Read the model definition and answer for the solid it produces. Units are mm, in the model's axes. A direction names the side the tool comes from. Give positions to 0.01 mm unless a question says otherwise; leave off trailing zeros. Order: outer loops, then holes, each group sorted by start corner. A loop starts at its lowest first (then second) coordinate and runs counter-clockwise, first axis right, second up. Notation, with made-up numbers: (58.5, 23.25) - (87.5, 23.25) arc R16 cw to (87.5, 37.25) - close; hole circle Ø3 at (85.25, 78.5). An arc over 180 degrees is marked (long way). Return JSON: item names as keys, results as strings.
Autodesk Inventor part; units mm, degrees
ref_plane "YZ Plane" through (0, 0, 0) normal (1, 0, 0) x (0, 1, 0)
ref_plane "XZ Plane" through (0, 0, 0) normal (0, 1, 0) x (-1, 0, 0)
ref_plane "XY Plane" through (0, 0, 0) normal (0, 0, 1) x (1, 0, 0)
sketch "스케치1" plane through (0, 0, 0) normal (0, 0, 1) x (1, 0, 0)
  line L0 (15, -15) -> (-15, -15)
  line L1 (-15, -15) -> (-15, 15)
  line L2 (-15, 15) -> (15, 15)
  line L3 (15, 15) -> (15, -15)
  circle A0 centre (0, 0) radius 2.5
  line L4 (-3.15, -15) -> (3.15, -15)
  line L5 (-4.15, -15) -> (4.15, -15)
  line L6 (3.15, -15) -> (3.15, -12.5)
  line L7 (-3.15, -12.5) -> (-3.15, -15)
  line L8 (-5.5, -12.5) -> (5.5, -12.5)
  line L9 (5.5, -12.5) -> (5.5, -6.9)
  line L10 (-5.5, -6.9) -> (-5.5, -12.5)
  line L11 (-5.5, -6.9) -> (-3, -4.4)
  line L12 (5.5, -6.9) -> (3, -4.4)
  line L13 (-3, -4.4) -> (3, -4.4)
  line L14 (-13.25, -13.25) -> (-7.25, -13.25)
  line L15 (-7.25, -13.25) -> (-7.25, -7.25)
  line L16 (-7.25, -7.25) -> (-13.25, -7.25)
  line L17 (-13.25, -7.25) -> (-13.25, -13.25)
  line L18 (0, 0) -> (-1, 0)
  line L19 (0, 0) -> (0, -1)
  line L20 (13.25, -13.25) -> (7.25, -13.25)
  line L21 (7.25, -13.25) -> (7.25, -7.25)
  line L22 (7.25, -7.25) -> (13.25, -7.25)
  line L23 (13.25, -7.25) -> (13.25, -13.25)
  line L24 (-13.25, 13.25) -> (-7.25, 13.25)
  line L25 (-7.25, 13.25) -> (-7.25, 7.25)
  line L26 (-7.25, 7.25) -> (-13.25, 7.25)
  line L27 (-13.25, 7.25) -> (-13.25, 13.25)
  line L28 (13.25, 7.25) -> (13.25, 13.25)
  line L29 (13.25, 13.25) -> (7.25, 13.25)
  line L30 (7.25, 13.25) -> (7.25, 7.25)
  line L31 (7.25, 7.25) -> (13.25, 7.25)
  line L32 (6.9, 5.5) -> (4.4, 3)
  line L33 (12.5, 5.5) -> (6.9, 5.5)
  line L34 (15, -3.15) -> (15, 3.15)
  line L35 (15, -4.15) -> (15, 4.15)
  line L36 (15, 3.15) -> (12.5, 3.15)
  line L37 (12.5, -3.15) -> (15, -3.15)
  line L38 (12.5, -5.5) -> (12.5, 5.5)
  line L39 (6.9, -5.5) -> (12.5, -5.5)
  line L40 (4.4, -3) -> (4.4, 3)
  line L41 (6.9, -5.5) -> (4.4, -3)
  line L42 (-5.5, 6.9) -> (-3, 4.4)
  line L43 (-5.5, 12.5) -> (-5.5, 6.9)
  line L44 (3.15, 15) -> (-3.15, 15)
  line L45 (4.15, 15) -> (-4.15, 15)
  line L46 (-3.15, 15) -> (-3.15, 12.5)
  line L47 (3.15, 12.5) -> (3.15, 15)
  line L48 (5.5, 12.5) -> (-5.5, 12.5)
  line L49 (5.5, 6.9) -> (5.5, 12.5)
  line L50 (3, 4.4) -> (-3, 4.4)
  line L51 (5.5, 6.9) -> (3, 4.4)
  line L52 (-6.9, -5.5) -> (-4.4, -3)
  line L53 (-12.5, -5.5) -> (-6.9, -5.5)
  line L54 (-15, 3.15) -> (-15, -3.15)
  line L55 (-15, 4.15) -> (-15, -4.15)
  line L56 (-15, -3.15) -> (-12.5, -3.15)
  line L57 (-12.5, 3.15) -> (-15, 3.15)
  line L58 (-12.5, 5.5) -> (-12.5, -5.5)
  line L59 (-6.9, 5.5) -> (-12.5, 5.5)
  line L60 (-4.4, 3) -> (-4.4, -3)
  line L61 (-6.9, 5.5) -> (-4.4, 3)
  dimension "d0" = 30
  dimension "d1" = 30
  dimension "d4" = 6.3
  dimension "d20" = 6
  dimension "d21" = 6
  dimension "d22" = 1
  dimension "d23" = 1
  dimension "d26" = 360
extrude "돌출1" add sketch "스케치1" along normal blind 144.5 contours L0 L6 L8 L9 L12 L13 L11 L10 L7 L1 L56 L58 L53 L52 L60 L61 L59 L57 L2 L46 L48 L43 L42 L50 L51 L49 L47 L3 L36 L38 L33 L32 L40 L41 L39 L37
properties part number "profile" material "알루미늄 6061"
Q1. Given pin 1 (4.5 mm diameter, centred on x = 0, y = 0, fed in from +Z), flat-ended and moving along its own axis, determine where the tip first touches the part or whether it passes through.
Values:
{"pin 1": "passes through"}
Q2. Consider L1, parallel to Y at x = -9.5, z = 7; L2, parallel to Y at x = 0, z = 65. Determine where each line is inside the solid, lowest interval first.
Values:
{"L1": "y = -15 to -13.25, -7.25 to -5.5, 5.5 to 7.25, 13.25 to 15", "L2": "y = -4.4 to -2.5, 2.5 to 4.4"}
Q3. A cutting plane is placed at B-B (x = 0). Write down the section's boundary in (y, z).
Values:
{"outline": "(-4.4, 0) - (-2.5, 0) - (-2.5, 144.5) - (-4.4, 144.5) - close; (2.5, 0) - (4.4, 0) - (4.4, 144.5) - (2.5, 144.5) - close"}
Q4. For faces 1 (the flat face through (3.15, -14, 71)), 2 (the flat face through (-4.4, 0, 71)), 3 (the flat face through (12.5, 4, 71)), determine the directions among +Z, -Z, +X, -X, +Y, -Y from which every point of the face is accessible in a straight line to the end or side of a thin tool.
Values:
{"face 1": "+Z, -Z, -Y", "face 2": "+Z, -Z, -X", "face 3": "+Z, -Z"}
Q5. A cutting plane is placed at A-A (y = -11.25). Write down the section's boundary in (x, z), and give its area (3 significant figures).
Values:
{"outline": "(-15, 0) - (-13.25, 0) - (-13.25, 144.5) - (-15, 144.5) - close; (-7.25, 0) - (-5.5, 0) - (-5.5, 144.5) - (-7.25, 144.5) - close; (5.5, 0) - (7.25, 0) - (7.25, 144.5) - (5.5, 144.5) - close; (13.25, 0) - (15, 0) - (15, 144.5) - (13.25, 144.5) - close", "area": "1,010 mm²"}
Q6. Determine the mould class of faces 4 (the flat face through (15, -9, 71)), 5 (the flat face through (4, -12.5, 71)), 6 (the flat face through (0, 4.4, 71)) for opening direction Y: released by +Y, released by -Y, zero draft, split by the parting line, or undercut.
Values:
{"face 4": "zero draft", "face 5": "undercut", "face 6": "released by +Y"}
